The listing builds one solid part. Answer for the finished solid, in the listing's coordinates (mm). A direction names the side the tool comes from. Give positions to 0.01 mm unless a question says otherwise; leave off trailing zeros. Order: outer loops, then holes, each group sorted by start corner. A loop starts at its lowest first (then second) coordinate and runs counter-clockwise, first axis right, second up. Notation, with made-up numbers: (69, 71) - (98, 71) arc R19 cw to (98, 104) - close; hole circle Ø5 at (-37, -8.75). An arc over 180 degrees is marked (long way). Use a Markdown table: item, result. Add a question column.
1) Find section B-B, the plane y = 21. Determine the outline of the cut face in (x, z).
2) The mould has two halves that part along X. Classify faces 6 (the face through (-21, 60, 0)), 7 (the face through (-20, 31, -10)), 8 (the face through (-36.79, 52.38, -7.07)), 9 (the face through (-21, 15, 0)): released by +X, released by -X, zero draft, split by the parting line, or undercut.
3) Straight lines are drawn through the part: line 1 (Z direction, x = -38.85, y = 45); line 2 (Z direction, x = -16, y = 59.5); line 3 (X direction, y = 9, z = 8.5). For each, find the intervals that lie inside material, in ascending order.
4) Find section C-C, the plane z = 3. Determine the outline of the cut face in (x, y), plus the area to 3 significant figures.
5) Flat-ended cylindrical pins translate along their axes: pin 1 (1.2 mm diameter, centred on x = -16.5, z = 0, fed in from +Y); pin 2 (12 mm diameter, centred on y = 14.5, z = -5, fed in from -X); pin 3 (12 mm diameter, centred on y = 48, z = -4, fed in from +X). Find the tip coordinate at first contact, or state that the pin passes through.
6) Find section D-D, the plane y = 32. Determine the outline of the cut face in (x, z).
7) Find section A-A, the plane y = 10. Determine the outline of the cut face in (x, z).
8) For faces 1 (the face through (-9.65, 3.41, -0.07)), 2 (the face through (-38.19, 45.35, -4.56)), 3 (the face through (-10.4, 0, 0.1)), 4 (the face through (-15.73, 57.44, -5.78)), 5 (the face through (-6, 43, 0)), determine the directions among +Z, -Z, +X, -X, +Y, -Y from which every point of the face is accessible in a straight line to the end or side of a thin tool.
from build123d import *

# Parameters (mm, degrees)
SKETCH1_R             = 2.5
BOSS_EXTRUDE1_DEPTH   = 10
CUT_EXTRUDE1_DEPTH    = 75.458041876
CUT_EXTRUDE2_DEPTH    = 2
M3_TAPPED_HOLE1_D     = 2.5
M3_TAPPED_HOLE1_DEPTH = 9
M3_TAPPED_HOLE1_TIP   = 0.751075774
SKETCH6_R             = 4
CUT_EXTRUDE3_DEPTH    = 75.458041876
SKETCH10_R            = 1.6
CUT_EXTRUDE4_DEPTH    = 8
SKETCH11_R            = 2
CUT_EXTRUDE5_DEPTH    = 20
SKETCH12_R            = 1
CUT_EXTRUDE6_DEPTH    = 29


# Read off the part's stored shape, not the designer's step: M4 Tapped Hole1
with BuildPart() as part:
    # Sketch1 → Boss-Extrude1 (new, symmetric)
    with BuildSketch(Plane.XY):
        Polygon((0, 0), (-21, 0), (-21, 30), (-40, 30), (-40, 62), (-12, 62), (0, 24), align=None)
        with Locations((-8, 20)):
            Circle(SKETCH1_R, mode=Mode.SUBTRACT)
    extrude(amount=BOSS_EXTRUDE1_DEPTH, both=True)

    # Sketch2 → Cut-Extrude1 (cut, through all)
    with BuildSketch(Plane(origin=(0, 62, 0), x_dir=(1, 0, 0), z_dir=(0, 1, 0))):
        with BuildLine():
            ThreePointArc((-23.291796068, -2), (-23.073333142, -1.010587075), (-23, 0))
            Line((-23, 0), (-37, 0))
            ThreePointArc((-37, 0), (-31.010587075, -6.926666858), (-23.291796068, -2))
        make_face()
        with BuildLine():
            Line((-37, 0), (-23, 0))
            ThreePointArc((-23, 0), (-23.073333142, 1.010587075), (-23.291796068, 2))
            ThreePointArc((-23.291796068, 2), (-31.010587075, 6.926666858), (-37, 0))
        make_face()
    extrude(amount=-CUT_EXTRUDE1_DEPTH, mode=Mode.SUBTRACT)

    # Sketch2<3> → Cut-Extrude2 (cut)
    with BuildSketch(Plane(origin=(0, 62, 0), x_dir=(1, 0, 0), z_dir=(0, 1, 0))):
        with BuildLine():
            ThreePointArc((-16, -2), (-17.414213562, -1.414213562), (-18, 0))
            Line((-18, 0), (-23, 0))
            ThreePointArc((-23, 0), (-23.073333142, -1.010587075), (-23.291796068, -2))
            Line((-23.291796068, -2), (-16, -2))
        make_face()
        with BuildLine():
            Line((-23, 0), (-18, 0))
            ThreePointArc((-18, 0), (-17.414213562, 1.414213562), (-16, 2))
            Line((-16, 2), (-23.291796068, 2))
            ThreePointArc((-23.291796068, 2), (-23.073333142, 1.010587075), (-23, 0))
        make_face()
        with BuildLine():
            ThreePointArc((-16, -2), (-14.585786438, -1.414213562), (-14, 0))
            Line((-14, 0), (-18, 0))
            ThreePointArc((-18, 0), (-17.414213562, -1.414213562), (-16, -2))
        make_face()
        with BuildLine():
            Line((-18, 0), (-14, 0))
            ThreePointArc((-14, 0), (-14.585786438, 1.414213562), (-16, 2))
            ThreePointArc((-16, 2), (-17.414213562, 1.414213562), (-18, 0))
        make_face()
    extrude(amount=-CUT_EXTRUDE2_DEPTH, mode=Mode.SUBTRACT)

    # M3 Tapped Hole1
    with Locations(Plane(origin=(0, 62, 0), x_dir=(1, 0, 0), z_dir=(0, 1, 0))):
        with Locations((-37, 7), (-37, -7), (-16, -7), (-16, 7)):
            Hole(M3_TAPPED_HOLE1_D / 2, depth=M3_TAPPED_HOLE1_DEPTH)
            with Locations((0, 0, -(M3_TAPPED_HOLE1_DEPTH + M3_TAPPED_HOLE1_TIP / 2))):  # 118° drill point
                Cone(0, M3_TAPPED_HOLE1_D / 2, M3_TAPPED_HOLE1_TIP, mode=Mode.SUBTRACT)

    # Sketch6 → Cut-Extrude3 (cut, through all)
    with BuildSketch(Plane(origin=(0, 0, 0), x_dir=(0, 0, -1), z_dir=(1, 0, 0))):
        with Locations(Location((0, 10, 0), (0, 0, 90))):
            Circle(SKETCH6_R)
    extrude(amount=-CUT_EXTRUDE3_DEPTH, mode=Mode.SUBTRACT)

    # M4 Tapped Hole1 outline → M4 Tapped Hole1 (revolve, cut)
    with BuildSketch(Plane(origin=(-16, 0, 0), x_dir=(1, 0, 0), z_dir=(0, 0, 1))):
        Polygon((1.65, 0.375), (1.65, 6.356330866), (0, 6.356330866), (0, 0), (2.025, 0), align=None)
    revolve(axis=Axis((-16, 0, 0), (0, 1, 0)), mode=Mode.SUBTRACT)

    # M4 Tapped Hole1 2 outline → M4 Tapped Hole1 2 (revolve, cut)
    with BuildSketch(Plane(origin=(-8, 0, 0), x_dir=(1, 0, 0), z_dir=(0, 0, 1))):
        Polygon((1.65, 0.375), (1.65, 6.356330866), (0, 6.356330866), (0, 0), (2.025, 0), align=None)
    revolve(axis=Axis((-8, 0, 0), (0, 1, 0)), mode=Mode.SUBTRACT)

    # Sketch10 → Cut-Extrude4 (cut)
    with BuildSketch(Plane.ZY.offset(40)):
        with Locations(Location((-3, 45, 0), (0, 0, 270))):
            Circle(SKETCH10_R)
        with Locations(Location((3, 45, 0), (0, 0, 270))):
            Circle(SKETCH10_R)
    extrude(amount=-CUT_EXTRUDE4_DEPTH, mode=Mode.SUBTRACT)

    # Sketch11 → Cut-Extrude5 (cut)
    with BuildSketch(Plane(origin=(0, 60, 0), x_dir=(1, 0, 0), z_dir=(0, 1, 0))):
        with Locations(Location((-16.005152977, 0, 0), (0, 0, 270))):
            Circle(SKETCH11_R)
    extrude(amount=-CUT_EXTRUDE5_DEPTH, mode=Mode.SUBTRACT)

    # Sketch12 → Cut-Extrude6 (cut)
    with BuildSketch(Plane(origin=(0, 40, 0), x_dir=(1, 0, 0), z_dir=(0, 1, 0))):
        with Locations(Location((-16, 0, 0), (0, 0, 270))):
            Circle(SKETCH12_R)
    extrude(amount=-CUT_EXTRUDE6_DEPTH, mode=Mode.SUBTRACT)


solid = part.part
The answers:
| question | item | result |
|---|---|---|
| 1 | outline | (-21, -10) - (-10.29, -10) - (-10.29, 10) - (-21, 10) - close; (-5.71, -10) - (0, -10) - (0, 10) - (-5.71, 10) - close; hole circle Ø2 at (-16, 0) |
| 2 | face 6 | undercut |
| 2 | face 7 | zero draft |
| 2 | face 8 | undercut |
| 2 | face 9 | released by -X |
| 3 | line 1 | -10 to -4.6, -1.4 to 1.4, 4.6 to 10 |
| 3 | line 2 | -10 to -8.25, -5.75 to -2, 2 to 5.75, 8.25 to 10 |
| 3 | line 3 | -21 to 0 |
| 4 | outline | (-40, 30) - (-36.32, 30) - (-36.32, 43.4) - (-40, 43.4) - close; (-40, 46.6) - (-36.32, 46.6) - (-36.32, 62) - (-40, 62) - close; (-23.68, 30) - (-21, 30) - (-21, 12.65) - (0, 12.65) - (0, 24) - (-12, 62) - (-23.68, 62) - close; (-21, 0) - (0, 0) - (0, 7.35) - (-21, 7.35) - close; hole circle Ø5 at (-8, 20) |
| 4 | area | 1,130 mm2 |
| 5 | pin 1 | y = 40 |
| 5 | pin 2 | x = -21 |
| 5 | pin 3 | x = -5.68 |
| 6 | outline | (-40, -10) - (-2.53, -10) - (-2.53, 10) - (-40, 10) - close; hole circle Ø14 at (-30, 0); hole circle Ø2 at (-16, 0) |
| 7 | outline | (-21, -10) - (0, -10) - (0, -4) - (-21, -4) - close; (-21, 4) - (0, 4) - (0, 10) - (-21, 10) - close |
| 8 | face 1 | -Y |
| 8 | face 2 | -X |
| 8 | face 3 | +Z, -Z, +X, -X, -Y |
| 8 | face 4 | +Y |
| 8 | face 5 | +Z, -Z, +X, +Y |
